from build123d import *

# Parameters (mm, degrees)
F1_DEPTH       = 2
F2_R           = 2
F2_R_2         = 0.9
F3_DEPTH       = 2
F5_D           = 1.8
F5_CBORE_D     = 4
F5_CBORE_DEPTH = 1.5


# Not quite as in the source:
# - after a boolean that leaves OpenCascade's solid faulty, fix() repairs it


with BuildPart() as f1:
    # F0 (on Front) → F1 (new body)
    with BuildSketch(Plane.XZ):
        with BuildLine():
            ThreePointArc((1.7320509844, 47.5114831651), (1.769e-07, 48.5114831651), (-1.7320506307, 47.5114831651))
            Line((-1.7320506307, 47.5114831651), (-41.9318474004, -22.1166072941))
            ThreePointArc((-41.9318474004, -22.1166072941), (-41.9318474004, -24.1166072941), (-40.1997965929, -25.1166072941))
            Line((-40.1997965929, -25.1166072941), (40.1997969466, -25.1166072941))
            ThreePointArc((40.1997969466, -25.1166072941), (41.9318477542, -24.1166072941), (41.9318477542, -22.1166072941))
            Line((41.9318477542, -22.1166072941), (1.7320509844, 47.5114831651))
        make_face()
        with BuildLine():
            ThreePointArc((-1.7320506307, 31.5114831651), (1.769e-07, 32.5114831651), (1.7320509844, 31.5114831651))
            Line((1.7320509844, 31.5114831651), (28.0754412936, -14.1166072941))
            ThreePointArc((28.0754412936, -14.1166072941), (28.0754412936, -16.1166072941), (26.343390486, -17.1166072941))
            Line((26.343390486, -17.1166072941), (-26.3433901323, -17.1166072941))
            ThreePointArc((-26.3433901323, -17.1166072941), (-28.0754409399, -16.1166072941), (-28.0754409399, -14.1166072941))
            Line((-28.0754409399, -14.1166072941), (-1.7320506307, 31.5114831651))
        make_face(mode=Mode.SUBTRACT)
    extrude(amount=F1_DEPTH)

    # F2 (on face) → F3 (join)
    with BuildSketch(Plane(origin=(0, 0, 0), x_dir=(-1, 0, 0), z_dir=(0, 1, 0))):
        with Locations((-1.769e-07, 40.5114831651)):
            Circle(F2_R)
        with Locations((-1.769e-07, 40.5114831651)):
            Circle(F2_R_2, mode=Mode.SUBTRACT)
        with Locations((-35.0036445239, -20.1166072941)):
            Circle(F2_R)
        with Locations((-35.0036445239, -20.1166072941)):
            Circle(F2_R_2, mode=Mode.SUBTRACT)
        with Locations((35.0036441701, -20.1166072941)):
            Circle(F2_R)
        with Locations((35.0036441701, -20.1166072941)):
            Circle(F2_R_2, mode=Mode.SUBTRACT)
    extrude(amount=F3_DEPTH)

    # F5 (through all)
    with Locations(Plane.XZ.offset(2)):
        with Locations((1.769e-07, 40.5114831651), (-35.0036441701, -20.1166072941), (35.0036445239, -20.1166072941)):
            CounterBoreHole(F5_D / 2, F5_CBORE_D / 2, F5_CBORE_DEPTH)

    add(f1.part.fix(), mode=Mode.REPLACE)


solid = f1.part
Verification items for the finished model (mm, model axes). A direction names the side the tool comes from. Give positions to 0.01 mm unless a question says otherwise; leave off trailing zeros. Order: outer loops, then holes, each group sorted by start corner. A loop starts at its lowest first (then second) coordinate and runs counter-clockwise, first axis right, second up. Notation, with made-up numbers: M -30.5,25.25 L 27.5,25.25 A25 ccw 27.5,55.25 Z; hole C 7.5,78.5 d2. An arc over 180 degrees is marked long. Use one line per item in the form item = value. Start each with the question number.
Q1. Mould release check, pull along Z, two halves, no side actions. Record for faces 4 (the flat face through (-1, 2, 40)), 5 (the flat face through (1, -0.5, 40)), 6 (the flat face through (-1, -1, -25.117)), 7 (the cylindrical face through (-0.03, -0.99, 32.51)): +Z half, -Z half, draft (parallel to the pull), parting line (faces both ways), or undercut.
Q2. Scan lines: line 1 along X through (y, z) = (0.1, 40.5); line 2 along Y through (x, z) = (1, 36.5); line 3 along Z through (x, y) = (23, -0.85). Record each from-to range of solid material in increasing order. Write a range as [from, to].
Q3. Go/stop test with flat-tipped pins: pin 1 Ø1.2 at (x, z) = (34, -20) entering from -Y; pin 2 Ø1 at (x, y) = (-10.5, -1) entering from +Z; pin 3 Ø1 at (y, z) = (-1, 29.5) entering from +X. Record where each tip stops, or that it passes through.
Q4. Section check B-B (z = 3.5). Enter the section's corners in (x, y).
Q5. Access from +Z, -Z, +X, -X, +Y, -Y to the whole of each face (thin tool, end or side, straight path). Record for faces 1 (the flat face through (-34, -0.5, -21)), 2 (the cylindrical face through (-28.06, -0.99, -16.14)), 3 (the cylindrical face through (0.26, 0.986, 42.494)).
Q6. Section check A-A (x = 0). Enter the section's corners in (y, z), then the cut area to 3 significant figures.
Q7. Section check D-D (z = 37). Enter the section's corners in (x, y).
Q8. Section check C-C (x = -25). Enter the section's corners in (y, z).
Evaluation:
q1.face_4 = draft
q1.face_5 = undercut
q1.face_6 = -Z half
q1.face_7 = undercut
q2.line_1 = [-2, -0.9], [0.9, 2]
q2.line_2 = [-2, 0]
q2.line_3 = [-25.12, -17.12], [-5.33, 10.67]
q3.pin_1 = -0.5
q3.pin_2 = 33.19
q3.pin_3 = 12.42
q4.outline = M -27.14,-2 L -17.9,-2 L -17.9,0 L -27.14,0 Z; M 17.9,-2 L 27.14,-2 L 27.14,0 L 17.9,0 Z
q5.face_1 = -Y
q5.face_2 = +Y, -Y
q5.face_3 = +Y
q6.outline = M -2,-25.12 L 0,-25.12 L 0,-17.12 L -2,-17.12 Z; M -2,32.51 L 0,32.51 L 0,38.51 L 2,38.51 L 2,39.61 L -0.5,39.61 L -0.5,38.51 L -2,38.51 Z; M -2,42.51 L -0.5,42.51 L -0.5,41.41 L 2,41.41 L 2,42.51 L 0,42.51 L 0,48.51 L -2,48.51 Z
q6.area = 45.5 mm2
q7.outline = M -7.8,-2 L 7.8,-2 L 7.8,0 L -7.8,0 Z
q8.outline = M -2,-25.12 L 0,-25.12 L 0,-17.12 L -2,-17.12 Z; M -2,-8.79 L 0,-8.79 L 0,7.21 L -2,7.21 Z
